Build history of the part. All positions in model axes, mm. A direction names the side the tool comes from. Give positions to 0.01 mm unless a question says otherwise; leave off trailing zeros. Write each loop counter-clockwise with the first axis right and the second up, starting at its lowest first coordinate (ties: lowest second). Pieces come first, ordered by that corner, then holes. Notation, with made-up numbers: (77.5, 64.5) -> (84.5, 64.5) arc R19 cw to (84.5, 72.5) -> close; hole circle Ø10 at (24, 37.5). An arc over 180 degrees is marked (long way). Put each result on its own line as item: value. Start each with the question number.
Item 1: Two-plate mould, pull along X, no slides. Class faces 5 (the flat face through (-56.25, 1, 15)), 6 (the flat face through (56.25, 1, 7)), 7 (the flat face through (-11, 2, -17.5)), 8 (the flat face through (-13.85, 2, 30)): pulls with the +X half, pulls with the -X half, needs draft (parallel to the pull), parting line crosses it, or undercut.
Item 2: Flat gauge pins, fed straight in: pin 1 Ø3 at (x, z) = (4, -10.5) entering from +Y; pin 2 Ø1.5 at (x, y) = (18.5, 1) entering from +Z; pin 3 Ø0.9 at (x, y) = (52, 1) entering from +Z; pin 4 Ø1.3 at (y, z) = (2, -14) entering from -X. Where does each tip first touch, or does it go through?
Item 3: Slice it at C-C, the plane z = 13.25. List the corners of the cut face in (x, y), plus the area to 3 significant figures.
Item 4: Slice it at D-D, the plane y = 1.9. Give the number of separate pieces and of enclosed holes in the cut face, plus the area to 3 significant figures.
Item 5: Slice it at B-B, the plane z = 30. List the corners of the cut face in (x, y).
Item 6: Drill centre lines: line 1 along X through (y, z) = (2.05, 2); line 2 along X through (y, z) = (1.85, 31); line 3 along X through (y, z) = (2.4, 20). Where is each one in solid material? Low to high.
Item 7: Tool access for faces 1 (the flat face through (-52, 2, -9.8)), 2 (the flat face through (53, 2, 23.25)), 3 (the cylindrical face through (14.42, 1.52, 32.65)), 4 (the flat face through (52, 2, -9.8)): list every direction of +Z, -Z, +X, -X, +Y, -Y with a clear straight run to the whole face (end or side of a thin tool).
Item 8: Slice it at A-A, the plane x = 18.5. List the corners of the cut face in (y, z), plus the area to 3 significant figures.
Autodesk Inventor part; units mm, degrees
ref_plane "YZ Plane" through (0, 0, 0) normal (1, 0, 0) x (0, 1, 0)
ref_plane "XZ Plane" through (0, 0, 0) normal (0, 1, 0) x (-1, 0, 0)
ref_plane "XY Plane" through (0, 0, 0) normal (0, 0, 1) x (1, 0, 0)
sketch "Sketch1" plane through (0, 0, 0) normal (0, 1, 0) x (-1, 0, 0)
  line L0 (-56.25, 58.25) -> (56.25, 58.25)
  line L1 (56.25, 58.25) -> (56.25, -58.25)
  line L2 (56.25, -58.25) -> (-56.25, -58.25)
  line L3 (-56.25, -58.25) -> (-56.25, 58.25)
  line L4 (-56.25, 58.25) -> (56.25, -58.25) construction
  line L5 (56.25, 58.25) -> (-56.25, -58.25) construction
  point P0 (0, 0)
  dimension "d0" = 112.5
  dimension "d1" = 116.5
extrude "Extrusion1" add sketch "Sketch1" along normal blind 3
sketch "Sketch2" plane through (0, 3, 0) normal (0, 1, 0) x (1, 0, 0)
  circle A0 centre (18.5, 28) radius 23.85
  circle A1 centre (37, -23.25) radius 13.85
  circle A2 centre (-35, -38.75) radius 13.85
  circle A3 centre (-30.9, 25.8) radius 13.85
  circle A4 centre (0, -23.25) radius 13.85
  line L0 (56.25, 58.25) -> (-56.25, 58.25)
  line L1 (-56.25, -58.25) -> (56.25, -58.25)
  line L2 (0, -105.9299) -> (0, 123.2086) construction
  line L3 (-76.4777, -38.75) -> (-5.35, -38.75) construction
  line L4 (-123.5447, -23.25) -> (82.5572, -23.25) construction
  line L5 (56.25, -58.25) -> (56.25, 58.25) construction
  point P0 (0, 0)
  dimension "d4" = 47.7
  dimension "d5" = 27.7
  dimension "d6" = 27.7
  dimension "d7" = 27.7
  dimension "d8" = 27.7
  dimension "d9" = 116.5
  dimension "d10" = 112.5
  dimension "d13" = 37
  dimension "d14" = 18.5
  dimension "d15" = 30.9
  dimension "d18" = 19.5
  dimension "d19" = 35
  dimension "d20" = 35
  dimension "d57" = 25.8
  dimension "d58" = 28
  dimension "d59" = 23.25
extrude "Extrusion2" cut sketch "Sketch2" against normal blind 5
sketch "Sketch3" plane through (0, 3, 0) normal (0, 1, 0) x (1, 0, 0)
  line L0 (-56.25, 58.25) -> (-56.25, -58.25)
  line L1 (56.25, -58.25) -> (56.25, 58.25)
  line L2 (18.5, -17.4904) -> (18.5, -40.0394) construction
  line L3 (-51.55, 5.4) -> (-51.55, 71.9941) construction
  line L4 (50.75, 5.4) -> (50.75, 69.4565) construction
  line L5 (-73.722, 50) -> (66.5467, 50) construction
  line L6 (66.5467, 30) -> (-76.0779, 30) construction
  circle A0 centre (18.5, 28) radius 23.85
  circle A1 centre (37, -23.25) radius 13.85
  circle A2 centre (-30.9, 25.8) radius 13.85
  circle A3 centre (0, -23.25) radius 13.85
  circle A4 centre (-35, -38.75) radius 13.85
  line L7 (56.25, 58.25) -> (-56.25, 58.25)
  line L8 (-56.25, 58.25) -> (-56.25, -58.25)
  line L9 (-56.25, -58.25) -> (56.25, -58.25)
  line L10 (56.25, -58.25) -> (56.25, 58.25)
  circle A5 centre (-30.9, 25.8) radius 13.85
  circle A6 centre (18.5, 28) radius 23.85
  circle A7 centre (0, -23.25) radius 13.85
  circle A8 centre (37, -23.25) radius 13.85
  circle A9 centre (-35, -38.75) radius 13.85
  line L11 (-56.25, 58.25) -> (-56.25, -58.25)
  line L12 (-56.25, 58.25) -> (-56.25, -58.25)
  line L13 (56.25, -58.25) -> (56.25, 58.25)
  line L14 (56.25, 58.25) -> (56.25, -58.25)
  line L15 (-56.25, 17.5) -> (-41.9875, 17.5)
  line L16 (-19.8125, 17.5) -> (-2.9143, 17.5)
  line L17 (39.1112, 16) -> (56.25, 16)
  line L18 (-56.25, -38.75) -> (-48.85, -38.75)
  circle A10 centre (-35, -38.75) radius 13.85
  circle A11 centre (37, -23.25) radius 13.85
  line L19 (50.85, -23.25) -> (56.25, -23.25)
  circle A12 centre (0, -23.25) radius 13.85
  line L20 (-13.85, -23.25) -> (-13.85, -36.75)
  line L21 (-15.85, -38.75) -> (-21.15, -38.75)
  line L22 (13.85, -23.25) -> (13.85, -31.25)
  line L23 (15.85, -33.25) -> (21.15, -33.25)
  line L24 (23.15, -31.25) -> (23.15, -23.25)
  arc A13 (13.85, -31.25) -> (15.85, -33.25) centre (15.85, -31.25) ccw
  arc A14 (21.15, -33.25) -> (23.15, -31.25) centre (21.15, -31.25) ccw
  arc A15 (-15.85, -38.75) -> (-13.85, -36.75) centre (-15.85, -36.75) ccw
  point P0 (0, 0)
  point P1 (0, 0)
  point P2 (18.5, -13.25)
  point P3 (18.5, -23.25)
  point P4 (-51.55, 50)
  point P5 (-51.55, 30)
  point P6 (50.75, 50)
  point P7 (50.75, 30)
  point P8 (-13.85, -38.75)
  point P9 (13.85, -33.25)
  point P10 (-2.9143, 17.5)
  point P11 (-56.25, -38.75)
  dimension "d21" = 4.7
  dimension "d22" = 5.5
  dimension "d23" = 13.25
  dimension "d24" = 30
  dimension "d25" = 50
  dimension "d26" = 5.4
  dimension "d27" = 5.4
  dimension "d29" = 18.5
  dimension "d31" = 10
  dimension "d32" = 2
  dimension "d55" = 27.7
  dimension "d56" = 47.7
  dimension "d60" = 2
  dimension "d61" = 27.7
  dimension "d62" = 23.25
  dimension "d63" = 37
  dimension "d64" = 17.5
  dimension "d65" = 17.5
  dimension "d66" = 16
hole "Hole1" at (-51.55, 3, -5.4) at (50.75, 3, -5.4) at (18.5, 3, 13.25) at (-51.55, 3, -50) at (-51.55, 3, -30) at (50.75, 3, -50) at (50.75, 3, -30) direction (0, -1, 0) diameter 4.2 end through all
extrude "Extrusion3" cut sketch "Sketch3" against normal blind 10 contours L7 L1 L17 A0 L16 A2 L15 L0 | L18 A4 L21 A15 L20 A3 L22 A13 L23 A14 L24 A1 L19 L1 L9 L0 | A3
sketch "Sketch4" plane through (0, 3, 0) normal (0, 1, 0) x (1, 0, 0)
  line L0 (-50.25, 75.9498) -> (-50.25, -88.0061) construction
  line L1 (-63.9145, -52.25) -> (79.4097, -52.25) construction
  line L2 (50.25, 66.2924) -> (50.25, -77.9097) construction
  line L3 (-56.25, 58.25) -> (-56.25, -58.25) construction
  line L4 (-56.25, -58.25) -> (56.25, -58.25) construction
  line L5 (56.25, -58.25) -> (56.25, 58.25) construction
  line L6 (-71.816, 40) -> (84.2384, 40) construction
  line L7 (-70.7185, 14) -> (79.4097, 14) construction
  line L8 (-56.25, 17.5) -> (-56.25, -38.75)
  line L9 (-56.25, 17.5) -> (-46.05, 17.5)
  line L10 (-46.05, 17.5) -> (-46.05, 12.8)
  line L11 (-49.05, 9.8) -> (-56.25, 9.8)
  line L12 (-56.25, 9.8) -> (-56.25, 17.5)
  line L13 (56.25, -23.25) -> (56.25, 16)
  line L14 (56.25, 16) -> (46.05, 16)
  line L15 (46.05, 16) -> (46.05, 12.8)
  line L16 (49.05, 9.8) -> (56.25, 9.8)
  line L17 (56.25, 9.8) -> (56.25, 16)
  line L18 (56.25, -23.25) -> (56.25, 16)
  line L19 (-56.25, 17.5) -> (-56.25, -38.75)
  arc A0 (-49.05, 9.8) -> (-46.05, 12.8) centre (-49.05, 12.8) ccw
  arc A1 (46.05, 12.8) -> (49.05, 9.8) centre (49.05, 12.8) ccw
  point P0 (0, 0)
  point P1 (0, 0)
  point P2 (-50.25, 40)
  point P3 (-50.25, 14)
  point P4 (-50.25, -52.25)
  point P5 (50.25, -52.25)
  point P6 (0, -52.25)
  point P7 (50.25, 14)
  point P8 (50.25, 40)
  dimension "d42" = 6
  dimension "d43" = 6
  dimension "d44" = 6
  dimension "d45" = 14
  dimension "d46" = 40
  dimension "d47" = 4.2
  dimension "d48" = 14
  dimension "d49" = 4.2
  dimension "d50" = 4.2
  dimension "d52" = 3
extrude "Extrusion4" cut sketch "Sketch4" against normal blind 10
fillet "Fillet1" radius 2 4 edges at (-56.25, 1.5, 38.75) (56.25, 1.5, 23.25) (56.25, 1.5, -9.8) (-56.25, 1.5, -9.8)
sketch "Sketch5" plane through (0, 3, 0) normal (0, 1, 0) x (1, 0, 0)
  point P0 (0, 0)
  point P1 (0, 0)
  point P2 (-34, -13)
  point P3 (-13, 11)
  point P4 (36, -2)
  dimension "d68" = 13
  dimension "d69" = 34
  dimension "d70" = 36
  dimension "d71" = 2
  dimension "d72" = 11
  dimension "d73" = 13
hole "Hole2" at (-34, 3, 13) at (-13, 3, -11) at (36, 3, 2) direction (0, -1, 0) diameter 3.2 end through all
fillet "Fillet2" radius 2 2 edges at (-46.05, 1.5, -17.5) (46.05, 1.5, -16)
properties part number "Bottle clamping plate 2"
Values follow:
1. face 5: pulls with the -X half
1. face 6: pulls with the +X half
1. face 7: needs draft
1. face 8: undercut
2. pin 1: y = 3
2. pin 2: z = 33.25
2. pin 3: z = 23.25
2. pin 4: x = -46.05
3. outline: (-56.25, 0) -> (-35.58, 0) -> (-35.58, 3) -> (-56.25, 3) -> close; (-32.42, 0) -> (-9.58, 0) -> (-9.58, 3) -> (-32.42, 3) -> close; (9.58, 0) -> (16.4, 0) -> (16.4, 3) -> (9.58, 3) -> close; (20.6, 0) -> (27.42, 0) -> (27.42, 3) -> (20.6, 3) -> close; (46.58, 0) -> (56.25, 0) -> (56.25, 3) -> (46.58, 3) -> close
3. area: 200 mm2
4. separate pieces: 1
4. enclosed holes: 6
4. area: 3,700 mm2
5. outline: (-56.25, 0) -> (-45.74, 0) -> (-45.74, 3) -> (-56.25, 3) -> close; (-24.26, 0) -> (-13.85, 0) -> (-13.85, 3) -> (-24.26, 3) -> close; (13.85, 0) -> (23.15, 0) -> (23.15, 3) -> (13.85, 3) -> close
6. line 1: -56.25 to 34.4, 37.6 to 56.25
6. line 2: -56.25 to -46.48, -23.52 to -13.85, 13.85 to 23.15
6. line 3: -56.25 to -13.46, 13.46 to 23.54, 50.46 to 56.25
7. face 1: -Z, -X, +Y, -Y
7. face 2: +Z, +X, +Y, -Y
7. face 3: +Z, +Y, -Y
7. face 4: -Z, +X, +Y, -Y
8. outline: (0, -4.15) -> (3, -4.15) -> (3, 11.15) -> (0, 11.15) -> close; (0, 15.35) -> (3, 15.35) -> (3, 33.25) -> (0, 33.25) -> close
8. area: 99.6 mm2
